For this review, take the finished solid that the model builds, in its own axes (mm). Coordinates: 2 decimals unless noted, no trailing zeros. Loops run counter-clockwise (first coordinate to the right, second up) from the corner with the lowest first, then second, coordinate; pieces in that order, holes last. Notation, with made-up numbers: (-33.5, 83.25) - (10.5, 83.25) arc R34 cw to (10.5, 119.25) - close; hole circle Ø11 at (22.25, 66.5). An arc over 180 degrees is marked (long way). Use one line per item in the form item = value. Start each with the question number.
1. Add section B-B on y = 27. Give the boundary of the cut face in (x, z), and give its area (3 significant figures).
2. Add section C-C on x = 37. Give the boundary of the cut face in (y, z), and give its area (3 significant figures).
3. Add section A-A on z = 8. Give the boundary of the cut face in (x, y).
4. Add section D-D on y = 19.05. Give the boundary of the cut face in (x, z), and give its area (3 significant figures).
5. To check wall thickness, follow probe 1 along X at (y, z) = (19, 14); probe 2 along X at (y, z) = (27.5, 15.5); probe 3 along Y at (x, z) = (13, 2). State the ranges of each line that lie inside material, in increasing order.
6. For pin 1 Ø4 at (y, z) = (28.5, 11) entering from -X; pin 2 Ø6.5 at (y, z) = (27, 14) entering from +X; pin 3 Ø2 at (x, z) = (-34.5, 24.5) entering from +Y, all flat-tipped, find the tip position at first contact; note any pin that passes through.
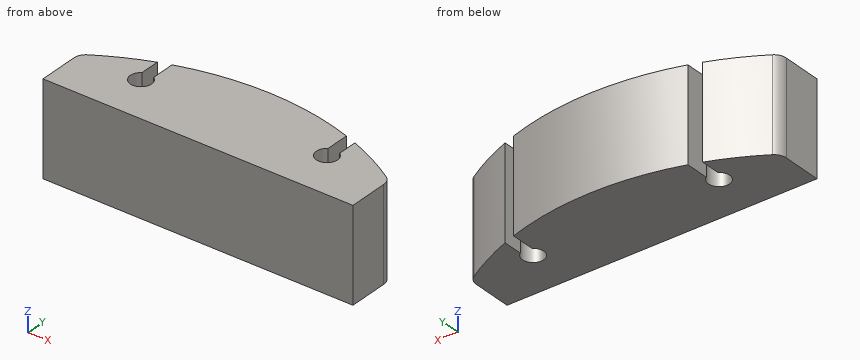
```python
from build123d import *

# Parameters (mm, degrees)
F1_DEPTH = 38.1
F2_R     = 5.08
F3_R     = 5.08


with BuildPart() as f1:
    # F0 (on Top) → F1 (new body)
    with BuildSketch(Plane.XY):
        with BuildLine():
            Line((-50.721363, 19.05), (-50.721363, 0))
            Line((-50.721363, 0), (76.278637, 0))
            Line((76.278637, 0), (76.278637, 19.05))
            ThreePointArc((76.278637, 19.05), (65.101151, 25.551684), (53.266237, 30.761569))
            Line((53.266237, 30.761569), (53.266237, 22.708658))
            ThreePointArc((53.266237, 22.708658), (50.878637, 14.6812), (48.491037, 22.708658))
            Line((48.491037, 22.708658), (48.491037, 32.432913))
            ThreePointArc((48.491037, 32.432913), (12.778637, 38.1), (-22.933763, 32.432913))
            Line((-22.933763, 32.432913), (-22.933763, 22.708658))
            ThreePointArc((-22.933763, 22.708658), (-25.321363, 14.6812), (-27.708963, 22.708658))
            Line((-27.708963, 22.708658), (-27.708963, 30.761569))
            ThreePointArc((-27.708963, 30.761569), (-39.543877, 25.551684), (-50.721363, 19.05))
        make_face()
    extrude(amount=F1_DEPTH)

    # F2
    f2_edges = [f1.edges().sort_by_distance(p)[0] for p in [
        (-50.721363, 19.05, 19.05),
    ]]
    fillet(f2_edges, radius=F2_R)

    # F3
    f3_edges = [f1.edges().sort_by_distance(p)[0] for p in [
        (76.278637, 19.05, 19.05),
    ]]
    fillet(f3_edges, radius=F3_R)


solid = f1.part
```
Conclusion:
q1.outline = (-36.59, 0) - (-27.71, 0) - (-27.71, 38.1) - (-36.59, 38.1) - close; (-22.93, 0) - (48.49, 0) - (48.49, 38.1) - (-22.93, 38.1) - close; (53.27, 0) - (62.15, 0) - (62.15, 38.1) - (53.27, 38.1) - close
q1.area = 3,400 mm^2
q2.outline = (0, 0) - (35.53, 0) - (35.53, 38.1) - (0, 38.1) - close
q2.area = 1,350 mm^2
q3.outline = (-50.72, 0) - (76.28, 0) - (76.28, 16.27) arc R5.08 ccw to (73.89, 20.58) arc R115.36 ccw to (53.27, 30.76) - (53.27, 22.71) arc R4.37 cw (long way) to (48.49, 22.71) - (48.49, 32.43) arc R115.36 ccw to (-22.93, 32.43) - (-22.93, 22.71) arc R4.37 cw (long way) to (-27.71, 22.71) - (-27.71, 30.76) arc R115.36 ccw to (-48.33, 20.58) arc R5.08 ccw to (-50.72, 16.27) - close
q4.outline = (-49.9, 0) - (-29.69, 0) - (-29.69, 38.1) - (-49.9, 38.1) - close; (-20.95, 0) - (46.51, 0) - (46.51, 38.1) - (-20.95, 38.1) - close; (55.25, 0) - (75.45, 0) - (75.45, 38.1) - (55.25, 38.1) - close
q4.area = 4,110 mm^2
q5.probe_1 = -49.93 to -29.69, -20.95 to 46.51, 55.25 to 75.49
q5.probe_2 = -35.52 to -27.71, -22.93 to 48.49, 53.27 to 61.08
q5.probe_3 = 0 to 38.1
q6.pin_1 = -37.64
q6.pin_2 = 68.5
q6.pin_3 = 28.41
